The listing builds one solid part. Answer for the finished solid, in the listing's coordinates (mm). Round coordinates to 2 decimals unless told otherwise and drop trailing zeros. Order: outer loops, then holes, each group sorted by start corner. A loop starts at its lowest first (then second) coordinate and runs counter-clockwise, first axis right, second up. Notation, with made-up numbers: (15, 65) - (34, 65) arc R7 ccw to (34, 75) - close; hole circle Ø7 at (53.5, 86). An arc over 180 degrees is marked (long way). One line per item, written item: value. Start each with the question number.
1. Section D-D, the plane z = 4.25 is taken. Count the separate pieces of the cut face and the enclosed holes in it, then the cut area to 3 significant figures.
2. Section B-B, the plane y = 57.15 is taken. Give the vertices of the cut face in (x, z).
3. Section A-A, the plane x = 31.75 is taken. Give the vertices of the cut face in (y, z), then the cut area to 3 significant figures.
4. Section C-C, the plane y = 97 is taken. Give the vertices of the cut face in (x, z).
5. Straight lines are drawn through the part: line 1 (Y direction, x = 19.05, z = 4.75); line 2 (Y direction, x = 59, z = 4.75); line 3 (X direction, y = 18, z = 1.75). For each, find the intervals that lie inside material, in ascending order.
6. Flat-ended cylindrical pins translate along their axes: P1, Ø5, axis at x = 51, y = 189.5, coming from the -Z side; P2, Ø5, axis at x = 57.15, y = 57.15, coming from the -Z side; P3, Ø2, axis at x = 59.5, z = 1.5, coming from the +Y side. Find the tip coordinate at first contact, or state that the pin passes through.
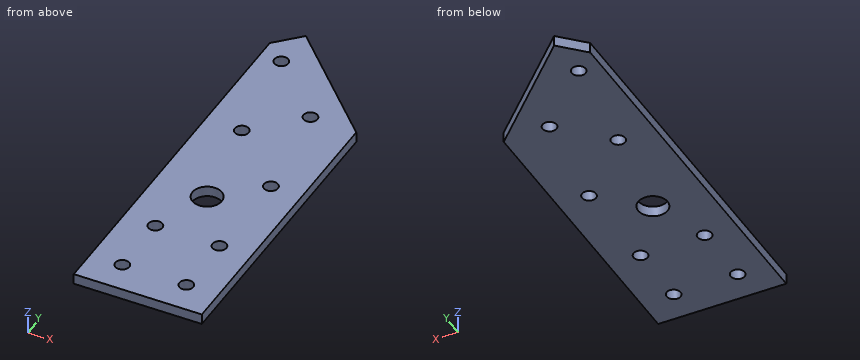
from build123d import *

# Parameters (mm, degrees)
BOSS_EXTRUDE1_DEPTH              = 6.35
F_21_64_0_32813_DIAMETER_HOLE1_D = 8.334502
LPATTERN1_COUNT                  = 2
LPATTERN1_PITCH                  = 38.1
LPATTERN1_COUNT_DIR2             = 2
LPATTERN1_PITCH_DIR2             = 38.1
F_21_64_0_32813_DIAMETER_HOLE2_D = 8.334502
LPATTERN2_COUNT                  = 3
LPATTERN2_PITCH                  = 50.8
LPATTERN2_COUNT_DIR2             = 2
LPATTERN2_PITCH_DIR2             = 38.1
F_11_16_0_6875_DIAMETER_HOLE1_D  = 17.4625


with BuildPart() as part:
    # Sketch1 → Boss-Extrude1 (new body)
    with BuildSketch(Plane.XY):
        Polygon((0, 0), (76.2, 0), (76.2, 177.8), (14.160193237, 239.839806763), (0, 225.679613527), align=None)
    extrude(amount=BOSS_EXTRUDE1_DEPTH)

    # 21/64 (0.32813) Diameter Hole1 (through all)
    with Locations(Plane.XY.offset(6.35)):
        with Locations((57.15, 19.05)):
            f_21_64_0_32813_diameter_hole1 = Hole(F_21_64_0_32813_DIAMETER_HOLE1_D / 2)

    # LPattern1: 21_64 _0.32813_ Diameter Hole1 2 × 2
    with Locations(*[(-i * LPATTERN1_PITCH, j * LPATTERN1_PITCH_DIR2, 0) for i in range(LPATTERN1_COUNT) for j in range(LPATTERN1_COUNT_DIR2) if (i, j) != (0, 0)]):
        add(f_21_64_0_32813_diameter_hole1, mode=Mode.SUBTRACT)

    # 21/64 (0.32813) Diameter Hole2 (through all)
    with Locations(Plane.XY.offset(6.35)):
        with Locations((12.7, 214.359231637)):
            f_21_64_0_32813_diameter_hole2 = Hole(F_21_64_0_32813_DIAMETER_HOLE2_D / 2)

    # LPattern2: 21_64 _0.32813_ Diameter Hole2 3 × 2, 2 skipped
    with Locations(*[Vector(0.7071067811865515, -0.7071067811865437, 0) * (i * LPATTERN2_PITCH) + Vector(-0.7071067811865441, -0.707106781186551, 0) * (j * LPATTERN2_PITCH_DIR2) for i in range(LPATTERN2_COUNT) for j in range(LPATTERN2_COUNT_DIR2) if (i, j) not in ((0, 0), (0, 1), (2, 0))]):
        add(f_21_64_0_32813_diameter_hole2, mode=Mode.SUBTRACT)

    # 11/16 (0.6875) Diameter Hole1 (through all)
    with Locations(Plane.XY.offset(6.35)):
        with Locations((31.75, 92.075)):
            Hole(F_11_16_0_6875_DIAMETER_HOLE1_D / 2)


solid = part.part
Answer list:
1. separate pieces: 1
1. enclosed holes: 9
1. area: 15,600 mm²
2. outline: (0, 0) - (14.88, 0) - (14.88, 6.35) - (0, 6.35) - close; (23.22, 0) - (52.98, 0) - (52.98, 6.35) - (23.22, 6.35) - close; (61.32, 0) - (76.2, 0) - (76.2, 6.35) - (61.32, 6.35) - close
3. outline: (0, 0) - (83.34, 0) - (83.34, 6.35) - (0, 6.35) - close; (100.81, 0) - (222.25, 0) - (222.25, 6.35) - (100.81, 6.35) - close
3. area: 1,300 mm²
4. outline: (0, 0) - (24.54, 0) - (24.54, 6.35) - (0, 6.35) - close; (38.96, 0) - (76.2, 0) - (76.2, 6.35) - (38.96, 6.35) - close
5. line 1: y = 0 to 14.88, 23.22 to 52.98, 61.32 to 148.27, 154.73 to 234.95
5. line 2: y = 0 to 15.32, 22.78 to 53.42, 60.88 to 111.65, 119.5 to 195
5. line 3: x = 0 to 15.02, 23.08 to 53.12, 61.18 to 76.2
6. P1: stops at z = 0
6. P2: passes through
6. P3: stops at y = 195.5
